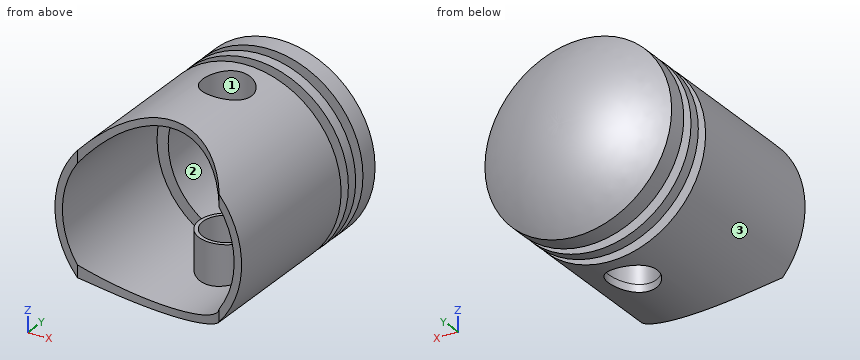
```python
from build123d import *

# Parameters (mm, degrees)
KES_EKSTR_ZYON1_DEPTH       = 25
KES_EKSTR_ZYON1_DEPTH_BACK  = 25
IZIM4_R                     = 6.5
KES_EKSTR_ZYON2_DEPTH       = 25
KES_EKSTR_ZYON2_DEPTH_BACK  = 25
Y_KSEKLIK_EKSTR_ZYON1_START = -23
IZIM5_R                     = 7.5
IZIM5_R_2                   = 6.5
Y_KSEKLIK_EKSTR_ZYON1_DEPTH = 11


with BuildPart() as part:
    # izim1 → D_nd_r39 (revolve)
    with BuildSketch(Plane.XY):
        with BuildLine():
            Line((-16.67359963, -12.856609108), (-16.67359963, 28.143390892))
            Line((-16.67359963, 28.143390892), (-13.67359963, 28.143390892))
            Line((-13.67359963, 28.143390892), (-13.67359963, 31.143390892))
            Line((-13.67359963, 31.143390892), (-16.67359963, 31.143390892))
            Line((-16.67359963, 31.143390892), (-16.67359963, 34.143390892))
            Line((-16.67359963, 34.143390892), (-13.67359963, 34.143390892))
            Line((-13.67359963, 34.143390892), (-13.67359963, 37.143390892))
            Line((-13.67359963, 37.143390892), (-16.67359963, 37.143390892))
            Line((-16.67359963, 37.143390892), (-16.67359963, 42.143390892))
            ThreePointArc((-16.67359963, 42.143390892), (-4.848501321, 48.252458677), (8.32640037, 50.143390892))
            Line((8.32640037, 50.143390892), (8.32640037, 48.143995987))
            Line((8.32640037, 48.143995987), (8.27720674, 48.143995987))
            ThreePointArc((8.27720674, 48.143995987), (-3.766624338, 46.495370879), (-14.67359963, 41.127902037))
            Line((-14.67359963, 41.127902037), (-14.67359963, 39.143390892))
            Line((-14.67359963, 39.143390892), (-11.67359963, 39.143390892))
            Line((-11.67359963, 39.143390892), (-11.67359963, 26.143390892))
            Line((-11.67359963, 26.143390892), (-14.67359963, 26.143390892))
            Line((-14.67359963, 26.143390892), (-14.67359963, -12.856609108))
            Line((-14.67359963, -12.856609108), (-16.67359963, -12.856609108))
        make_face()
    revolve(axis=Axis((8.32640037, 50.143390892, 0), (0, -1, 0)))

    # izim3 → Kes-Ekstr_zyon1 (cut, two sides)
    with BuildSketch(Plane.XY) as kes_ekstr_zyon1_sk:
        with BuildLine():
            Line((-10.67359963, -12.856609108), (27.32640037, -12.856609108))
            ThreePointArc((27.32640037, -12.856609108), (8.32640037, -2.856609108), (-10.67359963, -12.856609108))
        make_face()
    extrude(amount=KES_EKSTR_ZYON1_DEPTH, mode=Mode.SUBTRACT)
    extrude(kes_ekstr_zyon1_sk.sketch, amount=-KES_EKSTR_ZYON1_DEPTH_BACK, mode=Mode.SUBTRACT)

    # izim4 → Kes-Ekstr_zyon2 (cut, two sides)
    with BuildSketch(Plane.XY) as kes_ekstr_zyon2_sk:
        with Locations((9.310272977, 18.155492789)):
            Circle(IZIM4_R)
    extrude(amount=KES_EKSTR_ZYON2_DEPTH, mode=Mode.SUBTRACT)
    extrude(kes_ekstr_zyon2_sk.sketch, amount=-KES_EKSTR_ZYON2_DEPTH_BACK, mode=Mode.SUBTRACT)

    # izim5 → Y_kseklik-Ekstr_zyon1 (add)
    with BuildSketch(Plane.XY.offset(Y_KSEKLIK_EKSTR_ZYON1_START)):
        with Locations((9.310272977, 18.155492789)):
            Circle(IZIM5_R)
        with Locations((9.310272977, 18.155492789)):
            Circle(IZIM5_R_2, mode=Mode.SUBTRACT)
    y_kseklik_ekstr_zyon1 = extrude(amount=Y_KSEKLIK_EKSTR_ZYON1_DEPTH)

    # Aynalama1: Y_kseklik-Ekstr_zyon1 across plane
    add(y_kseklik_ekstr_zyon1.mirror(Plane.XY))


solid = part.part
```
Verification items for the finished model (mm, model axes). Face numbers are marked on the shaded views. Round coordinates to 2 decimals unless told otherwise and drop trailing zeros. Order: outer loops, then holes, each group sorted by start corner. A loop starts at its lowest first (then second) coordinate and runs counter-clockwise, first axis right, second up.
1) Cross-section at A-A, the plane y = 20. Record the cut outline in (x, z), plus the area to 3 significant figures.
Geometry says:
outline: (2.04, -22.12) arc R23 cw to (2.04, 22.12) - (2.04, 12) - (3.08, 12) - (3.08, 24.44) arc R25 ccw to (3.08, -24.44) - (3.08, -12) - (2.04, -12) - close; (15.54, -23.94) arc R25 ccw to (15.54, 23.94) - (15.54, 12) - (16.58, 12) - (16.58, 21.47) arc R23 cw to (16.58, -21.47) - (16.58, -12) - (15.54, -12) - close
area: 292 mm2
2) Material ranges on line 1 (Y direction, x = 9, z = -13); line 2 (X direction, y = 40, z = 0); line 3 (Y direction, x = 8.5, z = -15.5), recorded low to high.
Geometry says:
line 1: y = 10.66 to 11.66, 24.65 to 25.65, 46.2 to 48.3
line 2: x = -16.67 to -14.67, 31.33 to 33.33
line 3: y = 10.7 to 11.71, 24.6 to 25.61, 45.27 to 47.43
3) Draft check along Z on the marked faces 1, 2 and 3. Enter one of: +Z half, -Z half, draft (parallel to the pull), parting line (faces both ways), or undercut.
Geometry says:
face 1: draft
face 2: undercut
face 3: parting line
4) Depth check by flat-ended pin: pin 1 (6 mm diameter, centred on x = 2.5, z = -15.5, fed in from -Y); pin 2 (25 mm diameter, centred on x = 8, z = -7.5, fed in from -Y); pin 3 (7.5 mm diameter, centred on x = 7.5, y = 15, fed in from +Z); pin 4 (2 mm diameter, centred on x = 0, y = 29, fed in from +Z). Enter the tip coordinate at first touch or a pass-through.
Geometry says:
pin 1: stops at y = 11.7
pin 2: stops at y = 10.66
pin 3: stops at z = 25
pin 4: stops at z = 23.75
5) Cross-section at B-B, the plane z = 14.5. Give the number of separate pieces and of enclosed holes in the cut face, plus the area to 3 significant figures.
Geometry says:
separate pieces: 2
enclosed holes: 1
area: 462 mm2
6) Cross-section at C-C, the plane y = 2. Record the cut outline in (x, z).
Geometry says:
outline: circle Ø50 at (8.33, 0); hole circle Ø46 at (8.33, 0)
